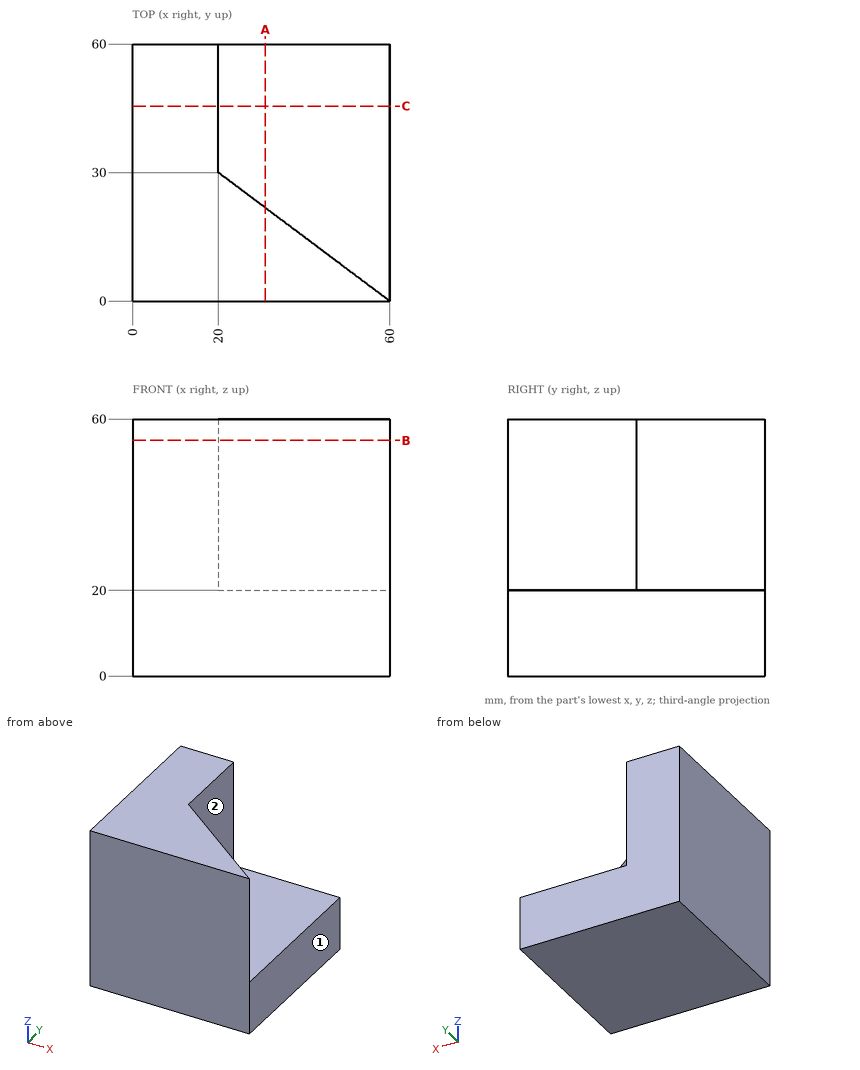
Part print with two shaded views. Sizes in mm from the minimum x, y, z corner. A direction names the side the tool comes from. Round coordinates to 2 decimals unless told otherwise and drop trailing zeros. Order: outer loops, then holes, each group sorted by start corner. A loop starts at its lowest first (then second) coordinate and runs counter-clockwise, first axis right, second up. Notation, with made-up numbers: M 3,26.25 L 51,26.25 A6 ccw 51,34.25 Z; hole C -34,28.25 d8. An arc over 180 degrees is marked long. Answer in a Markdown table with one row per item. Add a question column.
Q1. 3-axis set-ups, long thin cutter, end or side, ignore diameter. For the marked faces 1 and 2: which of +Z, -Z, +X, -X, +Y, -Y reach the whole face in a straight line?
Q2. Cut at B-B on z = 55. Give the cut face in (x, y), and give its area (3 significant figures).
Q3. Cut at C-C on y = 45.5. Give the cut face in (x, z), and give its area (3 significant figures).
Q4. Cut at A-A on x = 31. Give the cut face in (y, z).
Q5. Pin check, flat tips, straight feed: pin 1 (1 mm diameter, centred on x = 40, y = 22.5, fed in from +Z); pin 2 (9 mm diameter, centred on y = 50, z = 47.5, fed in from +X). Stop position of each tip, or through.
Q6. Wall check: L1, parallel to Z at x = 48, y = 43.5; L2, parallel to X at y = 20, z = 28. Give the ranges that are in metal, low to high. Write a range as from..to.
Established:
| question | item | result |
|---|---|---|
| 1 | face 1 | +Z, -Z, +X, +Y, -Y |
| 1 | face 2 | +Z, +X, +Y |
| 2 | outline | M 0,0 L 60,0 L 20,30 L 20,60 L 0,60 Z |
| 2 | area | 1,800 mm2 |
| 3 | outline | M 0,0 L 60,0 L 60,20 L 20,20 L 20,60 L 0,60 Z |
| 3 | area | 2,000 mm2 |
| 4 | outline | M 0,0 L 60,0 L 60,20 L 21.75,20 L 21.75,60 L 0,60 Z |
| 5 | pin 1 | stops at z = 20 |
| 5 | pin 2 | stops at x = 20 |
| 6 | L1 | z = 0..20 |
| 6 | L2 | x = 0..33.33 |
